The listing builds one solid part. Answer for the finished solid, in the listing's coordinates (mm). Coordinates: 2 decimals unless noted, no trailing zeros. Order: outer loops, then holes, each group sorted by start corner. A loop starts at its lowest first (then second) coordinate and runs counter-clockwise, first axis right, second up. Notation, with made-up numbers: (-32.75, 62.25) -> (-16.75, 62.25) arc R31 cw to (-16.75, 98.25) -> close; hole circle Ø3 at (-10, -39.75). An arc over 180 degrees is marked (long way). Return JSON: item names as keys, results as strings.
Autodesk Inventor part; units mm, degrees
ref_plane "YZ Plane" through (0, 0, 0) normal (1, 0, 0) x (0, 1, 0)
ref_plane "XZ Plane" through (0, 0, 0) normal (0, 1, 0) x (-1, 0, 0)
ref_plane "XY Plane" through (0, 0, 0) normal (0, 0, 1) x (1, 0, 0)
sketch "Sketch1" plane through (0, 0, 0) normal (0, 1, 0) x (-1, 0, 0)
  line L0 (381.1493, 61.7688) -> (30.4355, 61.7688)
  line L1 (380.945, 412.5458) -> (381.1493, 61.7688)
  line L2 (30.2312, 412.5458) -> (380.945, 412.5458)
  line L3 (30.4355, 61.7688) -> (30.4355, 412.5458)
  arc A0 (0.0979, 16.0688) -> (16.0979, 0.0688) centre (16.0979, 16.0688) ccw
  line L4 (0.1355, 16.0688) -> (-0.0688, 429.5458)
  arc A1 (15.9312, 445.5458) -> (-0.0688, 429.5458) centre (15.9312, 429.5458) ccw
  line L5 (15.9312, 445.5458) -> (395.245, 445.5458)
  arc A2 (411.245, 429.5458) -> (395.245, 445.5458) centre (395.245, 429.5458) ccw
  line L6 (411.245, 429.5458) -> (411.4493, 16.0688)
  arc A3 (395.4117, 0.0688) -> (411.4117, 16.0688) centre (395.4117, 16.0688) ccw
  line L7 (395.4117, 0.0688) -> (16.0979, 0.0688)
  arc A4 (21.3729, 6.5688) -> (25.1229, 6.5688) centre (23.2479, 6.5688) ccw
  line L8 (25.1229, 10.5688) -> (25.1229, 6.5688)
  arc A5 (25.1229, 10.5688) -> (21.3729, 10.5688) centre (23.2479, 10.5688) ccw
  line L9 (21.3729, 6.5688) -> (21.3729, 10.5688)
  arc A6 (52.3729, 6.5688) -> (56.1229, 6.5688) centre (54.2479, 6.5688) ccw
  line L10 (56.1229, 10.5688) -> (56.1229, 6.5688)
  arc A7 (56.1229, 10.5688) -> (52.3729, 10.5688) centre (54.2479, 10.5688) ccw
  line L11 (52.3729, 6.5688) -> (52.3729, 10.5688)
  arc A8 (21.3729, 37.5688) -> (25.1229, 37.5688) centre (23.2479, 37.5688) ccw
  line L12 (25.1229, 41.5688) -> (25.1229, 37.5688)
  arc A9 (25.1229, 41.5688) -> (21.3729, 41.5688) centre (23.2479, 41.5688) ccw
  line L13 (21.3729, 37.5688) -> (21.3729, 41.5688)
  arc A10 (52.3729, 37.5688) -> (56.1229, 37.5688) centre (54.2479, 37.5688) ccw
  line L14 (56.1229, 41.5688) -> (56.1229, 37.5688)
  arc A11 (56.1229, 41.5688) -> (52.3729, 41.5688) centre (54.2479, 41.5688) ccw
  line L15 (52.3729, 37.5688) -> (52.3729, 41.5688)
  arc A12 (26.7479, 22.0688) -> (50.7479, 22.0688) centre (38.7479, 22.0688) ccw
  line L16 (50.7479, 26.0688) -> (50.7479, 22.0688)
  arc A13 (50.7479, 26.0688) -> (26.7479, 26.0688) centre (38.7479, 26.0688) ccw
  line L17 (26.7479, 22.0688) -> (26.7479, 26.0688)
  arc A14 (355.4177, 6.5688) -> (359.1677, 6.5688) centre (357.2927, 6.5688) ccw
  line L18 (359.1677, 10.5688) -> (359.1677, 6.5688)
  arc A15 (359.1677, 10.5688) -> (355.4177, 10.5688) centre (357.2927, 10.5688) ccw
  line L19 (355.3867, 6.5688) -> (355.3867, 10.5688)
  arc A16 (386.3692, 6.5688) -> (390.1192, 6.5688) centre (388.2442, 6.5127) ccw
  arc A17 (386.3762, 37.5688) -> (390.1262, 37.5688) centre (388.2512, 37.5688) ccw
  line L20 (390.1262, 41.5688) -> (390.1262, 37.5688)
  arc A18 (390.1367, 41.5688) -> (386.3867, 41.5688) centre (388.2617, 41.5688) ccw
  line L21 (386.3762, 37.5688) -> (386.3762, 41.5688)
  arc A19 (355.3676, 37.5688) -> (359.1176, 37.5688) centre (357.2426, 37.5688) ccw
  line L22 (359.1176, 41.5688) -> (359.1176, 37.5688)
  arc A20 (359.1367, 41.5688) -> (355.3867, 41.5688) centre (357.2617, 41.5688) ccw
  line L23 (355.3676, 37.5688) -> (355.3676, 41.5688)
  arc A21 (360.7225, 22.0688) -> (384.7225, 22.0688) centre (372.7225, 22.0688) ccw
  line L24 (384.7225, 26.0688) -> (384.7225, 22.0688)
  arc A22 (384.7617, 26.0688) -> (360.7617, 26.0688) centre (372.7617, 26.0688) ccw
  line L25 (360.7225, 22.0688) -> (360.7225, 26.0688)
  circle A23 centre (50.1812, 420.5458) radius 2.1
  circle A24 centre (38.5812, 435.5458) radius 2.1
  circle A25 centre (372.595, 435.5458) radius 2.1
  circle A26 centre (360.995, 420.5458) radius 2.1
  circle A27 centre (25.8187, 418.0458) radius 1.6
  circle A28 centre (66.8187, 418.0458) radius 1.6
  circle A29 centre (205.5881, 418.0458) radius 1.6
  circle A30 centre (344.3575, 418.0458) radius 1.6
  circle A31 centre (385.3575, 418.0458) radius 1.6
  circle A32 centre (385.3575, 56.2688) radius 1
  circle A33 centre (344.3575, 56.2688) radius 1
  circle A34 centre (205.5881, 56.2688) radius 1
  circle A35 centre (66.8187, 56.2688) radius 1
  circle A36 centre (25.8187, 56.2688) radius 1
  arc A37 (390.1367, 10.5688) -> (386.3867, 10.5688) centre (388.2617, 10.5688) ccw
  line L26 (378.8577, 179.5323) -> (32.233, 179.5323)
  circle A38 centre (60.683, 222.8073) radius 1.6
  circle A39 centre (60.683, 258.6198) radius 1.6
  circle A40 centre (60.683, 186.9948) radius 1.6
  circle A41 centre (350.4077, 186.9948) radius 1.6
  circle A42 centre (350.4077, 222.8073) radius 1.6
  circle A43 centre (350.4077, 258.6198) radius 1.6
  circle A44 centre (49.883, 185.8823) radius 1.6
  circle A45 centre (49.883, 259.7323) radius 1.6
  circle A46 centre (361.2077, 222.8073) radius 1.6
  line L27 (378.8577, 266.0823) -> (378.8577, 179.5323)
  line L28 (345.9077, 256.5573) -> (345.9077, 189.0573)
  line L29 (65.183, 256.5573) -> (345.9077, 256.5573)
  line L30 (65.183, 189.0573) -> (65.183, 256.5573)
  line L31 (345.9077, 189.0573) -> (65.183, 189.0573)
  line L32 (32.233, 179.5323) -> (32.233, 266.0823)
  line L33 (32.233, 266.0823) -> (378.8577, 266.0823)
  circle A47 centre (50.183, 204.5073) radius 2.1
  circle A48 centre (360.9077, 204.5073) radius 2.1
  circle A49 centre (360.9077, 241.1073) radius 2.1
  circle A50 centre (50.183, 241.1073) radius 2.1
  line L34 (224.6381, 203.7573) -> (186.5381, 203.7573)
  line L35 (224.6381, 207.8163) -> (224.6381, 203.7573)
  arc A51 (226.0481, 209.3136) -> (224.6381, 207.8163) centre (226.1381, 207.8163) ccw
  arc A52 (226.0481, 209.3136) -> (226.0481, 216.301) centre (225.8381, 212.8073) ccw
  arc A53 (224.6381, 217.7983) -> (226.0481, 216.301) centre (226.1381, 217.7983) ccw
  arc A54 (226.0481, 229.3136) -> (224.6381, 227.8163) centre (226.1381, 227.8163) ccw
  arc A55 (226.0481, 229.3136) -> (226.0481, 236.301) centre (225.8381, 232.8073) ccw
  arc A56 (224.6381, 237.7983) -> (226.0481, 236.301) centre (226.1381, 237.7983) ccw
  line L36 (186.5381, 241.8573) -> (224.6381, 241.8573)
  line L37 (186.5381, 237.7983) -> (186.5381, 241.8573)
  arc A57 (185.1281, 236.301) -> (186.5381, 237.7983) centre (185.0381, 237.7983) ccw
  arc A58 (185.1281, 236.301) -> (185.1281, 229.3136) centre (185.3381, 232.8073) ccw
  arc A59 (186.5381, 227.8163) -> (185.1281, 229.3136) centre (185.0381, 227.8163) ccw
  arc A60 (185.1281, 216.301) -> (186.5381, 217.7983) centre (185.0381, 217.7983) ccw
  arc A61 (185.1281, 216.301) -> (185.1281, 209.3136) centre (185.3381, 212.8073) ccw
  arc A62 (186.5381, 207.8163) -> (185.1281, 209.3136) centre (185.0381, 207.8163) ccw
  line L38 (173.8381, 254.5573) -> (237.3381, 254.5573)
  line L39 (237.3381, 254.5573) -> (237.3381, 191.0573)
  line L40 (237.3381, 191.0573) -> (173.8381, 191.0573)
  line L41 (173.8381, 191.0573) -> (173.8381, 254.5573)
  circle A63 centre (180.1881, 196.9948) radius 0.875
  circle A64 centre (230.9881, 196.9948) radius 0.875
  circle A65 centre (230.9881, 248.6198) radius 0.875
  circle A66 centre (180.1881, 248.6198) radius 0.875
  circle A67 centre (177.8381, 232.8073) radius 0.875
  circle A68 centre (233.3381, 232.8073) radius 0.875
  circle A69 centre (233.3381, 212.8073) radius 0.875
  circle A70 centre (177.8381, 212.8073) radius 0.875
  line L42 (186.5381, 203.7573) -> (186.5381, 207.8163)
  line L43 (186.5381, 217.7983) -> (186.5381, 227.8163)
  line L44 (224.6381, 241.8573) -> (224.6381, 237.7983)
  line L45 (224.6381, 227.8163) -> (224.6381, 217.7983)
  line L46 (390.1367, 10.5688) -> (390.1367, 6.5605)
  line L47 (386.3867, 10.5688) -> (386.3867, 6.2509)
  circle A71 centre (136.8187, 56.2688) radius 1
  circle A72 centre (273.8511, 56.2688) radius 1
  circle A73 centre (274.3575, 418.0458) radius 1.6
  circle A74 centre (136.8187, 418.0458) radius 1.6
  point P0 (0, 0)
extrude "Extrusion1" add sketch "Sketch1" along normal blind 4 contours L26 L32 L33 L27
properties part number "300 mm core xy gantry"
1. The part is cut by section A-A on x = -228. Give the vertices of the cut face in (y, z).
Answer block:
{"outline": "(0, 179.53) -> (4, 179.53) -> (4, 189.06) -> (0, 189.06) -> close; (0, 256.56) -> (4, 256.56) -> (4, 266.08) -> (0, 266.08) -> close"}
2. Each of these flat-tipped pins is pushed along its axis until it touches: pin 1 Ø3 at (x, z) = (-60.68, 258.62) entering from +Y; pin 2 Ø4 at (x, z) = (-350.41, 258.62) entering from +Y. Where does it stop, or does it pass through?
Answer block:
{"pin 1": "passes through", "pin 2": "stops at y = 4"}
3. The part is cut by section C-C on y = 0.9. Give the number of separate pieces and of enclosed holes in the cut face, and give its area (3 significant figures).
Answer block:
{"separate pieces": "1", "enclosed holes": "14", "area": "10,900 mm2"}
4. The part is cut by section B-B on z = 193. Give the vertices of the cut face in (x, y), and give its area (3 significant figures).
Answer block:
{"outline": "(-378.86, 0) -> (-345.91, 0) -> (-345.91, 4) -> (-378.86, 4) -> close; (-65.18, 0) -> (-32.23, 0) -> (-32.23, 4) -> (-65.18, 4) -> close", "area": "264 mm2"}
5. Consider line 1 (X direction, y = 3.3, z = 204); line 2 (X direction, y = 3.85, z = 254); line 3 (Z direction, x = -224, y = 1.15). Determine where each line is inside the solid, lowest interval first. Write a range as from..to.
Answer block:
{"line 1": "x = -378.86..-362.95, -358.87..-345.91, -65.18..-52.22, -48.15..-32.23", "line 2": "x = -378.86..-345.91, -65.18..-32.23", "line 3": "z = 179.53..189.06, 256.56..266.08"}
